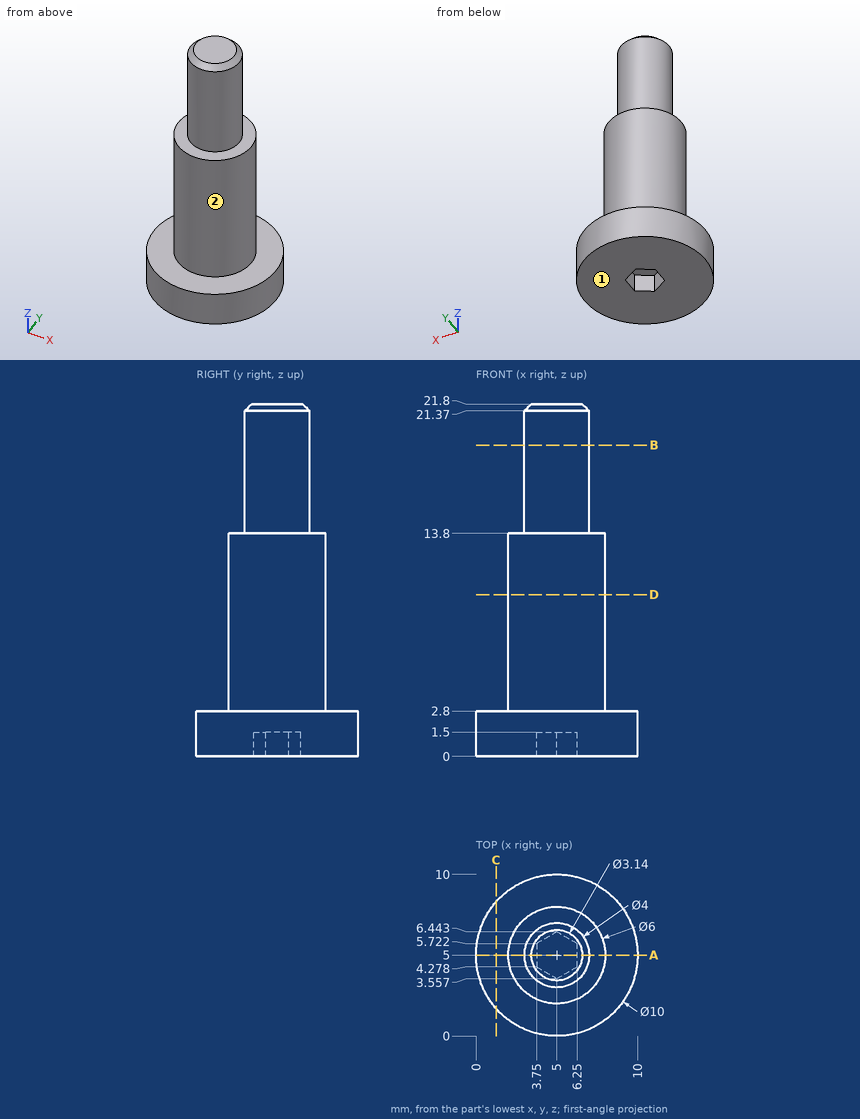
Here's the drawing with two shaded views (mm, measured from the low corner). I have some questions. A direction names the side the tool comes from. Coordinates: 2 decimals unless noted, no trailing zeros. Loops run counter-clockwise (first coordinate to the right, second up) from the corner with the lowest first, then second, coordinate; pieces in that order, holes last. Notation, with made-up numbers: (56.25, -6) -> (72.25, -6) arc R9 ccw to (72.25, 2) -> close; hole circle Ø7 at (71, 24). An arc over 180 degrees is marked (long way). Put each result on its own line as item: value. Start each with the question number.
Q1. I want a section at A-A (y = 5). Write out the boundary of the cut face in (x, z).
Q2. I want a section at B-B (z = 19.25). Write out the boundary of the cut face in (x, y), plus the area to 3 significant figures.
Q3. For the marked faces 1 and 2, which set-ups out of +Z, -Z, +X, -X, +Y, -Y let a thin tool reach every point of the face, with its end or its side?
Q4. I want a section at C-C (x = 1.25). Write out the boundary of the cut face in (y, z).
Q5. I'm going to push flat-ended pins straight in: P1, Ø5, axis at x = 5, z = 12.5, coming from the -Y side; P2, Ø2, axis at y = 5.5, z = 8.5, coming from the -X side; P3, Ø5, axis at x = 3, z = 15.5, coming from the +Y side (1 decimal). Where does each tip first touch, or does it pass through?
Q6. I want a section at D-D (z = 10). Write out the boundary of the cut face in (x, y).
Q7. If I drill on line 1 (Z direction, x = 4.5, y = 2.5); line 2 (Z direction, x = 4.25, y = 5.5); line 3 (Y direction, x = 5, z = 8), over which ranges is the centre line in solid material (lowest first)? Write a range as [from, to].
Taken from the geometry:
1. outline: (0, 0) -> (3.75, 0) -> (3.75, 1.5) -> (6.25, 1.5) -> (6.25, 0) -> (10, 0) -> (10, 2.8) -> (8, 2.8) -> (8, 13.8) -> (7, 13.8) -> (7, 21.37) -> (6.57, 21.8) -> (3.43, 21.8) -> (3, 21.37) -> (3, 13.8) -> (2, 13.8) -> (2, 2.8) -> (0, 2.8) -> close
2. outline: circle Ø4 at (5, 5)
2. area: 12.6 mm2
3. face 1: -Z, +X, -X, +Y, -Y
3. face 2: +Z
4. outline: (1.69, 0) -> (8.31, 0) -> (8.31, 2.8) -> (1.69, 2.8) -> close
5. P1: stops at y = 2
5. P2: stops at x = 2
5. P3: stops at y = 8
6. outline: circle Ø6 at (5, 5)
7. line 1: z = [0, 13.8]
7. line 2: z = [1.5, 21.8]
7. line 3: y = [2, 8]
